Check sheet for the modelled part. Datum: model origin and axes. Units: mm. Face numbers are marked on the shaded views. A direction names the side the tool comes from. Give positions to 0.01 mm unless a question says otherwise; leave off trailing zeros. Write each loop counter-clockwise with the first axis right and the second up, starting at its lowest first coordinate (ties: lowest second). Pieces come first, ordered by that corner, then holes. Notation, with made-up numbers: (-21, 31.25) - (11, 31.25) arc R23 ccw to (11, 55.25) - close; hole circle Ø6 at (17.25, 55.5). An arc over 180 degrees is marked (long way). Return JSON: item names as keys, results as strings. Group by question number.
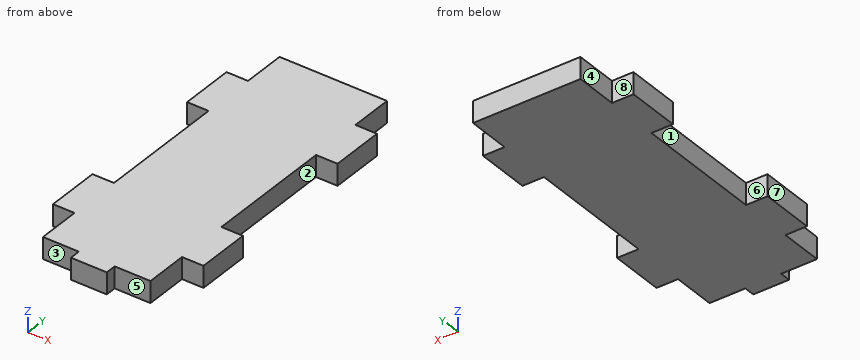
Autodesk Inventor part; units mm, degrees
ref_plane "YZ Plane" through (0, 0, 0) normal (1, 0, 0) x (0, 1, 0)
ref_plane "XZ Plane" through (0, 0, 0) normal (0, 1, 0) x (-1, 0, 0)
ref_plane "XY Plane" through (0, 0, 0) normal (0, 0, 1) x (1, 0, 0)
sketch "Boceto1" plane through (0, 0, 0) normal (0, 0, 1) x (1, 0, 0)
  line L0 (0, 0) -> (30, 0)
  line L1 (30, 0) -> (30, 90)
  line L2 (30, 90) -> (0, 90)
  line L3 (0, 90) -> (0, 0)
  line L4 (30, 78) -> (36, 78)
  line L5 (36, 78) -> (36, 63)
  line L6 (36, 63) -> (30, 63)
  line L7 (30, 63) -> (30, 78)
  line L8 (30, 45) -> (0, 45) construction
  line L9 (30, 12) -> (36, 12)
  line L10 (36, 12) -> (36, 27)
  line L11 (36, 27) -> (30, 27)
  line L12 (30, 27) -> (30, 12)
  line L13 (15, 90) -> (15, 45) construction
  line L14 (0, 78) -> (-6, 78)
  line L15 (-6, 78) -> (-6, 63)
  line L16 (-6, 63) -> (0, 63)
  line L17 (0, 63) -> (0, 78)
  line L18 (0, 12) -> (-6, 12)
  line L19 (-6, 12) -> (-6, 27)
  line L20 (-6, 27) -> (0, 27)
  line L21 (0, 27) -> (0, 12)
  point P0 (30, 12)
  point P1 (30, 27)
  point P2 (30, 63)
  dimension "d0" = 30
  dimension "d1" = 90
  dimension "d2" = 6
  dimension "d3" = 15
  dimension "d4" = 12
extrude "Extrusión1" add sketch "Boceto1" along normal blind 6
sketch "Boceto3" plane through (0, 0, 0) normal (0, -1, 0) x (1, 0, 0)
  line L0 (30, 6) -> (0, 6)
  line L1 (30, 0) -> (0, 0)
  line L2 (10, 6) -> (20, 6)
  line L3 (20, 6) -> (20, 0)
  line L4 (20, 0) -> (10, 0)
  line L5 (10, 0) -> (10, 6)
  point P0 (15, 6)
  point P1 (15, 6)
  dimension "d11" = 10
extrude "Extrusión3" add sketch "Boceto3" along normal blind 3
properties part number "Caja_CaraFrontal"
Item 1: Depth check by flat-ended pin: pin 1 (3 mm diameter, centred on x = 34.5, z = 3.5, fed in from +Y); pin 2 (3 mm diameter, centred on x = 34, z = 4.5, fed in from -Y); pin 3 (1 mm diameter, centred on x = 31.5, y = 56, fed in from +Z); pin 4 (2 mm diameter, centred on x = 18, y = 68.5, fed in from -Z). Enter the tip coordinate at first touch or a pass-through.
Item 2: Mould release check, pull along Y, two halves, no side actions. Record for the marked faces 6, 7 and 8: +Y half, -Y half, draft (parallel to the pull), parting line (faces both ways), or undercut.
Item 3: Section check A-A on x = 32. Record the cut outline in (y, z), plus the area to 3 significant figures.
Item 4: Section check C-C on x = 7.5. Record the cut outline in (y, z), plus the area to 3 significant figures.
Item 5: Section check D-D on y = 30.5. Record the cut outline in (x, z).
Item 6: Section check B-B on z = 4.15. Record the cut outline in (x, y), plus the area to 3 significant figures.
Item 7: Access from +Z, -Z, +X, -X, +Y, -Y to the whole of each face (thin tool, end or side, straight path). Record for the marked faces 1, 2, 3, 4 and 5.
Item 8: Material ranges on line 1 along Y through (x, z) = (33.5, 4.2); line 2 along Y through (x, z) = (4.5, 5.75); line 3 along X through (y, z) = (11, 2.9), recorded low to high. Write a range as from..to.
Reply:
{
 "1": {"pin 1": "y = 78", "pin 2": "y = 12", "pin 3": "through", "pin 4": "z = 0"},
 "2": {"face 6": "undercut", "face 7": "draft", "face 8": "+Y half"},
 "3": {"outline": "(12, 0) - (27, 0) - (27, 6) - (12, 6) - close; (63, 0) - (78, 0) - (78, 6) - (63, 6) - close", "area": "180 mm²"},
 "4": {"outline": "(0, 0) - (90, 0) - (90, 6) - (0, 6) - close", "area": "540 mm²"},
 "5": {"outline": "(0, 0) - (30, 0) - (30, 6) - (0, 6) - close"},
 "6": {"outline": "(-6, 12) - (0, 12) - (0, 0) - (10, 0) - (10, -3) - (20, -3) - (20, 0) - (30, 0) - (30, 12) - (36, 12) - (36, 27) - (30, 27) - (30, 63) - (36, 63) - (36, 78) - (30, 78) - (30, 90) - (0, 90) - (0, 78) - (-6, 78) - (-6, 63) - (0, 63) - (0, 27) - (-6, 27) - close", "area": "3,090 mm²"},
 "7": {"face 1": "+Z, -Z, -X", "face 2": "+Z, -Z, +X", "face 3": "+Z, -Z, -X, -Y", "face 4": "+Z, -Z, -X, +Y", "face 5": "+Z, -Z, +X, -Y"},
 "8": {"line 1": "12..27, 63..78", "line 2": "0..90", "line 3": "0..30"}
}
